CAD build for the part. Positions are in the model's coordinates, mm. Coordinates: 2 decimals unless noted, no trailing zeros. Loops run counter-clockwise (first coordinate to the right, second up) from the corner with the lowest first, then second, coordinate; pieces in that order, holes last.
1) Saw through at A-A, the plane x = 9. Write the cut outline in (y, z).
2) Two-plate mould, pull along X, no slides. Class faces 1 (the flat face through (-17, -5, 0)), 2 (the cylindrical face through (23.15, 0.09, 9.86)), 3 (the cylindrical face through (-18.85, 0.09, 9.86)), 4 (the cylindrical face through (23.846, 7.509, 9.86)): +X half, -X half, draft (parallel to the pull), parting line (faces both ways), or undercut.
3) Saw through at B-B, the plane y = -15. Write the cut outline in (x, z), and give its area (3 significant figures).
4) Wall check: line 1 along X through (y, z) = (-0.5, 18) (3 decimals); line 2 along Y through (x, z) = (10.5, 10.75); line 3 along X through (y, z) = (1.5, 6.5). Give the ranges that are in metal, low to high.
5) Saw through at C-C, the plane x = -5. Write the cut outline in (y, z), and give its area (3 significant figures).
6) Saw through at D-D, the plane y = -1.5. Write the cut outline in (x, z), and give its area (3 significant figures).
7) Pin check, flat tips, straight feed: pin 1 Ø3.5 at (x, y) = (10.5, 18.19) entering from +Z; pin 2 Ø4 at (x, z) = (1.5, 9.5) entering from -Y; pin 3 Ø3 at (y, z) = (-13.5, 5.5) entering from +X; pin 4 Ø5 at (x, z) = (-13, 12.5) entering from -Y. Stop position of each tip, or through.
```python
from build123d import *

# Parameters (mm, degrees)
CROQUIS1_R                   = 25
CROQUIS1_R_2                 = 17.5
SALIENTE_EXTRUIR1_DEPTH      = 20
TALADRO_DE_MARGEN_PARA_M41_D = 4.3


with BuildPart() as part:
    # Croquis1 → Saliente-Extruir1 (new body)
    with BuildSketch(Plane.XY):
        Circle(CROQUIS1_R)
        Circle(CROQUIS1_R_2, mode=Mode.SUBTRACT)
    extrude(amount=SALIENTE_EXTRUIR1_DEPTH)

    # Taladro de margen para M41 (through all)
    with Locations(Plane.XY.offset(20)):
        with Locations((21, 0), (10.5, -18.186533479), (-10.5, -18.186533479), (-21, 0), (-10.5, 18.186533479), (10.5, 18.186533479)):
            Hole(TALADRO_DE_MARGEN_PARA_M41_D / 2)


solid = part.part
```
Data:
1. outline: (-23.32, 0) - (-19.73, 0) - (-19.73, 20) - (-23.32, 20) - close; (-16.65, 0) - (-15.01, 0) - (-15.01, 20) - (-16.65, 20) - close; (15.01, 0) - (16.65, 0) - (16.65, 20) - (15.01, 20) - close; (19.73, 0) - (23.32, 0) - (23.32, 20) - (19.73, 20) - close
2. face 1: draft
2. face 2: undercut
2. face 3: undercut
2. face 4: parting line
3. outline: (-20, 0) - (-9.01, 0) - (-9.01, 20) - (-20, 20) - close; (9.01, 0) - (20, 0) - (20, 20) - (9.01, 20) - close
3. area: 439 mm2
4. line 1: x = -24.995 to -23.091, -18.909 to -17.493, 17.493 to 18.909, 23.091 to 24.995
4. line 2: y = -22.69 to -20.34, -16.04 to -14, 14 to 16.04, 20.34 to 22.69
4. line 3: x = -24.95 to -22.54, -19.46 to -17.44, 17.44 to 19.46, 22.54 to 24.95
5. outline: (-24.49, 0) - (-16.77, 0) - (-16.77, 20) - (-24.49, 20) - close; (16.77, 0) - (24.49, 0) - (24.49, 20) - (16.77, 20) - close
5. area: 309 mm2
6. outline: (-24.95, 0) - (-22.54, 0) - (-22.54, 20) - (-24.95, 20) - close; (-19.46, 0) - (-17.44, 0) - (-17.44, 20) - (-19.46, 20) - close; (17.44, 0) - (19.46, 0) - (19.46, 20) - (17.44, 20) - close; (22.54, 0) - (24.95, 0) - (24.95, 20) - (22.54, 20) - close
6. area: 178 mm2
7. pin 1: passes through
7. pin 2: stops at y = -25
7. pin 3: stops at x = 21.93
7. pin 4: stops at y = -22.69
